The model under review builds one solid part; all positions refer to its coordinate system, in mm. A direction names the side the tool comes from. Coordinates: 2 decimals unless noted, no trailing zeros. Order: outer loops, then holes, each group sorted by start corner. A loop starts at its lowest first (then second) coordinate and runs counter-clockwise, first axis right, second up. Notation, with made-up numbers: M 75,10 L 92,10 A21 ccw 92,33 Z; hole C 28.5,16.5 d7. An arc over 180 degrees is marked long. Answer in a Markdown table with one row per item.
from build123d import *

# Parameters (mm, degrees)
SKETCH1_W           = 5.9
SKETCH1_H           = 4.5
BOSS_EXTRUDE1_DEPTH = 6
SKETCH2_W           = 4.9
SKETCH2_H           = 3.5
CUT_EXTRUDE1_DEPTH  = 5.5
SKETCH3_W           = 1
SKETCH3_H           = 1.9
CUT_EXTRUDE2_DEPTH  = 0.5
BOSS_EXTRUDE2_START = -2.9
SKETCH4_W           = 0.5
SKETCH4_H           = 0.5
BOSS_EXTRUDE2_DEPTH = 7.9
SKETCH5_W           = 0.8
SKETCH5_H           = 2
CUT_EXTRUDE3_DEPTH  = 0.5
SKETCH6_W           = 0.8
SKETCH6_H           = 4
CUT_EXTRUDE4_DEPTH  = 0.5


with BuildPart() as part:
    # Sketch1 → Boss-Extrude1 (new body)
    with BuildSketch(Plane(origin=(0, 0, 0), x_dir=(1, 0, 0), z_dir=(0, 1, 0))):
        Rectangle(SKETCH1_W, SKETCH1_H)
    extrude(amount=BOSS_EXTRUDE1_DEPTH)

    # Sketch2 → Cut-Extrude1 (cut)
    with BuildSketch(Plane(origin=(0, 6, 0), x_dir=(1, 0, 0), z_dir=(0, 1, 0))):
        Rectangle(SKETCH2_W, SKETCH2_H)
    extrude(amount=-CUT_EXTRUDE1_DEPTH, mode=Mode.SUBTRACT)

    # Sketch3 → Cut-Extrude2 (cut)
    with BuildSketch(Plane.XY.offset(2.25)):
        with Locations((-1.95, 3.15)):
            Rectangle(SKETCH3_W, SKETCH3_H)
    cut_extrude2 = extrude(amount=-CUT_EXTRUDE2_DEPTH, mode=Mode.SUBTRACT)

    # Sketch4 → Boss-Extrude2 (add)
    with BuildSketch(Plane(origin=(0, 0.5, 0), x_dir=(1, 0, 0), z_dir=(0, 1, 0)).offset(BOSS_EXTRUDE2_START)):
        with Locations((-1, -0.55)):
            Rectangle(SKETCH4_W, SKETCH4_H)
    boss_extrude2 = extrude(amount=BOSS_EXTRUDE2_DEPTH)

    # Sketch5 → Cut-Extrude3 (cut)
    with BuildSketch(Plane.ZY.offset(2.95)):
        with Locations((0.55, 5)):
            Rectangle(SKETCH5_W, SKETCH5_H)
    cut_extrude3 = extrude(amount=-CUT_EXTRUDE3_DEPTH, mode=Mode.SUBTRACT)

    # Mirror1: Cut-Extrude2, Cut-Extrude3 across plane
    add(cut_extrude2.mirror(Plane(origin=(0, 0, 0), x_dir=(0, 0, 1), z_dir=(1, 0, 0))), mode=Mode.SUBTRACT)
    add(cut_extrude3.mirror(Plane(origin=(0, 0, 0), x_dir=(0, 0, 1), z_dir=(1, 0, 0))), mode=Mode.SUBTRACT)

    # Sketch6 → Cut-Extrude4 (cut)
    with BuildSketch(Plane.XY.offset(2.25)):
        with Locations((0, 4)):
            Rectangle(SKETCH6_W, SKETCH6_H)
    extrude(amount=-CUT_EXTRUDE4_DEPTH, mode=Mode.SUBTRACT)

    # Mirror2: Boss-Extrude2 across plane
    add(boss_extrude2.mirror(Plane(origin=(0, 0, 0), x_dir=(0, 0, 1), z_dir=(1, 0, 0))))


solid = part.part
(1) Take a section at C-C (x = -2.15). Write out the cut boundary in (y, z), then the cut area to 3 significant figures.
Report:
| item | result |
|---|---|
| outline | M 0,-2.25 L 6,-2.25 L 6,-1.75 L 0.5,-1.75 L 0.5,1.75 L 2.2,1.75 L 2.2,2.25 L 0,2.25 Z; M 4.1,1.75 L 6,1.75 L 6,2.25 L 4.1,2.25 Z |
| area | 6.80 mm^2 |
(2) Take a section at B-B (y = 3.75). Write out the cut boundary in (x, z), then the cut area to 3 significant figures.
Report:
| item | result |
|---|---|
| outline | M -2.95,-2.25 L 2.95,-2.25 L 2.95,2.25 L 2.45,2.25 L 2.45,-1.75 L -2.45,-1.75 L -2.45,2.25 L -2.95,2.25 Z; M -1.45,1.75 L -0.4,1.75 L -0.4,2.25 L -1.45,2.25 Z; M -1.25,0.3 L -0.75,0.3 L -0.75,0.8 L -1.25,0.8 Z; M 0.4,1.75 L 1.45,1.75 L 1.45,2.25 L 0.4,2.25 Z; M 0.75,0.3 L 1.25,0.3 L 1.25,0.8 L 0.75,0.8 Z |
| area | 8.50 mm^2 |
(3) Take a section at D-D (z = 2.05). Write out the cut boundary in (x, y), then the cut area to 3 significant figures.
Report:
| item | result |
|---|---|
| outline | M -2.95,0 L 2.95,0 L 2.95,6 L 0.4,6 L 0.4,2 L -0.4,2 L -0.4,6 L -2.95,6 Z; hole M -2.45,2.2 L -1.45,2.2 L -1.45,4.1 L -2.45,4.1 Z; hole M 1.45,2.2 L 2.45,2.2 L 2.45,4.1 L 1.45,4.1 Z |
| area | 28.4 mm^2 |
(4) Take a section at A-A (y = 1). Write out the cut boundary in (x, z), then the cut area to 3 significant figures.
Report:
| item | result |
|---|---|
| outline | M -2.95,-2.25 L 2.95,-2.25 L 2.95,2.25 L -2.95,2.25 Z; M -1.25,0.3 L -0.75,0.3 L -0.75,0.8 L -1.25,0.8 Z; M 0.75,0.3 L 1.25,0.3 L 1.25,0.8 L 0.75,0.8 Z; hole M -2.45,-1.75 L 2.45,-1.75 L 2.45,1.75 L -2.45,1.75 Z |
| area | 9.90 mm^2 |
(5) The part is to be moulded in two halves that separate along Z. For faces 3 (the flat face through (0, 3, -1.75)), 4 (the flat face through (-2.95, 3, 0)), 5 (the flat face through (0, 3, -2.25)), 6 (the flat face through (0, 0.5, 0)), say which applies: +Z half, -Z half, draft (parallel to the pull), parting line (faces both ways), or undercut.
Report:
| item | result |
|---|---|
| face 3 | undercut |
| face 4 | draft |
| face 5 | -Z half |
| face 6 | undercut |
(6) Machinability: for faces 1 (the flat face through (-1, 3, 1.75)), 2 (the flat face through (-1, 3, 2.25)), which of the approach directions +Z, -Z, +X, -X, +Y, -Y give a long, thin tool a straight path to every point of the face, cutting with its end or side? Answer none if there is none.
Report:
| item | result |
|---|---|
| face 1 | +Y |
| face 2 | +Z, +X, -X, +Y, -Y |
(7) To check wall thickness, follow line 1 (X direction, y = 2, z = -1.45); line 2 (X direction, y = -0.75, z = 0.5); line 3 (Z direction, x = -0.5, y = 1.25). State the ranges of each line that lie inside material, in increasing order. Write a range as [from, to].
Report:
| item | result |
|---|---|
| line 1 | [-2.95, -2.45], [2.45, 2.95] |
| line 2 | [-1.25, -0.75], [0.75, 1.25] |
| line 3 | [-2.25, -1.75], [1.75, 2.25] |
(8) Insertion check: P1, Ø1, axis at x = 2, z = 0, coming from the +Y side; P2, Ø0.6, axis at x = -2, z = 2, coming from the -Y side. Each pin has a flat end and moves straight along its axis. Give the tip position at first contact, or say it passes through.
Report:
| item | result |
|---|---|
| P1 | y = 6 |
| P2 | y = 0 |
